from build123d import *

# Parameters (mm, degrees)
SKETCH1_R               = 6
BOSS_EXTRUDE1_DEPTH     = 20
SKETCH2_R               = 3.4
CUT_EXTRUDE1_DEPTH      = 13.55
SKETCH5_W               = 1.550685087
SKETCH5_H               = 7.184215806
BOSS_EXTRUDE2_DEPTH     = 13.55
SKETCH7_W               = 18.003976239
SKETCH7_H               = 19.909960041
BOSS_EXTRUDE3_DEPTH     = 12
SKETCH6_R               = 2
CUT_EXTRUDE2_DEPTH      = 1
CUT_EXTRUDE2_DEPTH_BACK = 13.55
NUTOPENING_DEPTH        = 10
SKETCH10_R              = 50
BOSS_EXTRUDE4_DEPTH     = 30
SKETCH12_R              = 47.082764373
SKETCH12_R_2            = 15.95790089
CUT_EXTRUDE5_DEPTH      = 27
SKETCH13_R              = 50
SKETCH13_R_2            = 47.082764373
BOSS_EXTRUDE5_DEPTH     = 10
CUT_EXTRUDE6_DEPTH      = 6.933086
SKETCH16_R              = 7
CUT_EXTRUDE7_DEPTH      = 40


with BuildPart() as part:
    # Sketch1 → Boss-Extrude1 (new body)
    with BuildSketch(Plane(origin=(0, 0, 0), x_dir=(1, 0, 0), z_dir=(0, 1, 0))):
        Circle(SKETCH1_R)
    extrude(amount=BOSS_EXTRUDE1_DEPTH)

    # Sketch2 → Cut-Extrude1 (cut)
    with BuildSketch(Plane(origin=(0, 20, 0), x_dir=(1, 0, 0), z_dir=(0, 1, 0))):
        Circle(SKETCH2_R)
    extrude(amount=-CUT_EXTRUDE1_DEPTH, mode=Mode.SUBTRACT)

    # Sketch5 → Boss-Extrude2 (add)
    with BuildSketch(Plane(origin=(0, 18.26, 0), x_dir=(1, 0, 0), z_dir=(0, 1, 0))):
        with Locations((3.375342544, 0.020519704)):
            Rectangle(SKETCH5_W, SKETCH5_H)
    extrude(amount=-BOSS_EXTRUDE2_DEPTH)

    # Sketch7 → Boss-Extrude3 (add)
    with BuildSketch(Plane.ZY.offset(-2.6)):
        with Locations((0.33027221, 9.954980021)):
            Rectangle(SKETCH7_W, SKETCH7_H)
    extrude(amount=-BOSS_EXTRUDE3_DEPTH)

    # Sketch6 → Cut-Extrude2 (cut, two sides)
    with BuildSketch(Plane.ZY.offset(-2.6)) as cut_extrude2_sk:
        with Locations((0, 10.236925537)):
            Circle(SKETCH6_R)
    extrude(amount=CUT_EXTRUDE2_DEPTH, mode=Mode.SUBTRACT)
    extrude(cut_extrude2_sk.sketch, amount=-CUT_EXTRUDE2_DEPTH_BACK, mode=Mode.SUBTRACT)

    # Sketch9 → NutOpening (cut)
    with BuildSketch(Plane.XY):
        Polygon((11.876516377, 10.236925537), (11.876516377, 5.861925537), (4.943430227, 5.861925537), (4.943430227, 10.236925537), (4.943430227, 14.614332445), (11.876516377, 14.614332445), align=None)
    extrude(amount=-NUTOPENING_DEPTH, mode=Mode.SUBTRACT)

    # Sketch10 → Boss-Extrude4 (add)
    with BuildSketch(Plane.XZ):
        Circle(SKETCH10_R)
    extrude(amount=BOSS_EXTRUDE4_DEPTH)

    # Sketch12 → Cut-Extrude5 (cut)
    with BuildSketch(Plane(origin=(0, 0, 0), x_dir=(1, 0, 0), z_dir=(0, 1, 0))):
        Circle(SKETCH12_R)
        Circle(SKETCH12_R_2, mode=Mode.SUBTRACT)
    extrude(amount=-CUT_EXTRUDE5_DEPTH, mode=Mode.SUBTRACT)

    # Sketch13 → Boss-Extrude5 (add)
    with BuildSketch(Plane(origin=(0, 0, 0), x_dir=(1, 0, 0), z_dir=(0, 1, 0))):
        Circle(SKETCH13_R)
        Circle(SKETCH13_R_2, mode=Mode.SUBTRACT)
    extrude(amount=BOSS_EXTRUDE5_DEPTH)

    # Sketch14 → Cut-Extrude6 (cut)
    with BuildSketch(Plane.ZY.offset(-11.876516377)):
        Polygon((-5.054124256, 10.236925537), (-2.527062128, 5.859925537), (2.527062128, 5.859925537), (5.054124256, 10.236925537), (2.527062128, 14.613925537), (-2.527062128, 14.613925537), align=None)
    extrude(amount=CUT_EXTRUDE6_DEPTH, mode=Mode.SUBTRACT)

    # Sketch16 → Cut-Extrude7 (cut)
    with BuildSketch(Plane(origin=(14.6, 0, 0), x_dir=(0, 0, -1), z_dir=(1, 0, 0))):
        with Locations((0, 10.236925537)):
            Circle(SKETCH16_R)
    extrude(amount=CUT_EXTRUDE7_DEPTH, mode=Mode.SUBTRACT)


solid = part.part
Geometry: final body of the model. Coordinates: model frame, mm. A direction names the side the tool comes from. Give positions to 0.01 mm unless a question says otherwise; leave off trailing zeros. Write each loop counter-clockwise with the first axis right and the second up, starting at its lowest first coordinate (ties: lowest second). Pieces come first, ordered by that corner, then holes. Notation, with made-up numbers: (-2, -4.75) - (25, -4.75) arc R24 cw to (25, 26.25) - close; hole circle Ø3 at (-31.75, 80). An arc over 180 degrees is marked (long way). Return JSON: item names as keys, results as strings. Group by question number.
1) Section A-A on y = -24. Return the cut outline in (x, z), plus the area to 3 significant figures.
2) Set-up query: faces 4 (the flat face through (8, 5.86, 0)), 5 (the cylindrical face through (47.69, -10.28, -15.02)), 6 (the flat face through (3, 20, 3)), 7 (the flat face through (8, 14.614, -4)), 8 (the flat face through (2.6, 15, 0)). Return all of +Z, -Z, +X, -X, +Y, -Y with unobstructed straight access to the full face (end or side cutting, diameter ignored); none if empty.
3) First-contact query: P1, Ø1.2, axis at y = 11, z = 8.5, coming from the -X side; P2, Ø6.5, axis at x = -0.5, z = -1, coming from the +Y side; P3, Ø12, axis at y = 11, z = -11, coming from the +X side; P4, Ø8, axis at y = -3, z = -21.5, coming from the +X side. Flat tips, straight axial feed; report the tip coordinate or a pass-through.
4) Mould query, pull axis Y, two halves, no side actions, for faces 1 (the flat face through (-34, 10, 33)), 2 (the flat face through (14.6, 10.1, 2.2)), 3 (the flat face through (8, 14.614, 1)). Classes: released by +Y, released by -Y, zero draft, split by the parting line, or undercut.
5) Section C-C on z = 24.5. Return the cut outline in (x, y).
6) Section D-D on z = -29.5. Return the cut outline in (x, y).
7) Line query: line 1 (X direction, y = -3, z = 0); line 2 (Z direction, x = 0, y = 10.5). Output: solid intervals per line, ascending.
8) Section B-B on x = 0. Return the cut outline in (y, z), plus the area to 3 significant figures.
Filled in:
{
 "1": {"outline": "circle Ø100 at (0, 0); circle Ø31.92 at (0, 0); hole circle Ø94.17 at (0, 0)", "area": "1,690 mm^2"},
 "2": {"face 4": "none", "face 5": "+Y, -Y", "face 6": "+Z, -Z, +X, -X, +Y", "face 7": "-Z", "face 8": "+Y"},
 "3": {"P1": "stops at x = 2.6", "P2": "stops at y = 20", "P3": "stops at x = 49.6", "P4": "stops at x = 46.84"},
 "4": {"face 1": "released by +Y", "face 2": "zero draft", "face 3": "undercut"},
 "5": {"outline": "(-43.59, -30) - (43.59, -30) - (43.59, 10) - (40.21, 10) - (40.21, -27) - (-40.21, -27) - (-40.21, 10) - (-43.59, 10) - close"},
 "6": {"outline": "(-40.37, -30) - (40.37, -30) - (40.37, 10) - (36.7, 10) - (36.7, -27) - (-36.7, -27) - (-36.7, 10) - (-40.37, 10) - close"},
 "7": {"line 1": "x = -50 to -47.08, -15.96 to 15.96, 47.08 to 50", "line 2": "z = -6 to -3.4, 3.4 to 6"},
 "8": {"outline": "(-30, -50) - (10, -50) - (10, -47.08) - (-27, -47.08) - (-27, -15.96) - (0, -15.96) - (0, -6) - (20, -6) - (20, -3.4) - (6.45, -3.4) - (6.45, 3.4) - (20, 3.4) - (20, 6) - (0, 6) - (0, 15.96) - (-27, 15.96) - (-27, 47.08) - (10, 47.08) - (10, 50) - (-30, 50) - close", "area": "1,530 mm^2"}
}
